The listing builds one solid part. Answer for the finished solid, in the listing's coordinates (mm). A direction names the side the tool comes from. Round coordinates to 2 decimals unless told otherwise and drop trailing zeros. Write each loop counter-clockwise with the first axis right and the second up, starting at its lowest first coordinate (ties: lowest second). Pieces come first, ordered by that corner, then holes. Notation, with made-up numbers: (21.25, 32.25) - (45.25, 32.25) arc R5 ccw to (45.25, 38.25) - close; hole circle Ø2 at (48.5, 73). An arc over 180 degrees is marked (long way). Answer as CSV lines item,"result". Start each with the question number.
Item 1: Which of the six approach directions +Z, -Z, +X, -X, +Y, -Y give full straight-line access (tool end or side, diameter ignored) to faces 1 (the cylindrical face through (40.9, 15.5, 3)), 2 (the flat face through (18, -27.5, 3)), 3 (the cylindrical face through (180.9, -15.5, 3))?
Item 2: A cutting plane is placed at A-A on z = 3.8. State how many separate pieces and enclosed holes the cut face has, and give its area (3 significant figures).
Item 3: A flat-ended cylindrical pin translates along its axis: pin 1 (2 mm diameter, centred on x = 226, y = 0, fed in from -Z). Find the tip coordinate at first contact, or state that the pin passes through.
Item 4: A cutting plane is placed at B-B on x = 148.5. Determine the outline of the cut face in (y, z), and give its area (3 significant figures).
Item 5: Straight lines are drawn through the part: line 1 along Y through (x, z) = (15, 3.35); line 2 along Y through (x, z) = (38.5, 4.9); line 3 along X through (y, z) = (-11.5, 5.25). For each, find the intervals that lie inside material, in ascending order. Write a range as [from, to].
```python
from build123d import *

# Parameters (mm, degrees)
SKETCH1_W           = 240
SKETCH1_H           = 25
SKETCH1_R           = 1.75
BOSS_EXTRUDE1_DEPTH = 6
SKETCH2_W           = 50
SKETCH2_H           = 10
BOSS_EXTRUDE2_DEPTH = 6
SKETCH3_W           = 140
SKETCH3_H           = 4
CUT_EXTRUDE1_DEPTH  = 235.693949645
SKETCH4_R           = 2.75
CUT_EXTRUDE2_DEPTH  = 235.693949645
FILLET1_R           = 7


with BuildPart() as part:
    # Sketch1 → Boss-Extrude1 (new body)
    with BuildSketch(Plane.XY):
        with Locations((113, -5)):
            Rectangle(SKETCH1_W, SKETCH1_H)
        Circle(SKETCH1_R, mode=Mode.SUBTRACT)
        with Locations((226, 0)):
            Circle(SKETCH1_R, mode=Mode.SUBTRACT)
        with Locations((15, 0)):
            Circle(SKETCH1_R, mode=Mode.SUBTRACT)
        with Locations((0, -10)):
            Circle(SKETCH1_R, mode=Mode.SUBTRACT)
        with Locations((15, -10)):
            Circle(SKETCH1_R, mode=Mode.SUBTRACT)
        with Locations((211, 0)):
            Circle(SKETCH1_R, mode=Mode.SUBTRACT)
        with Locations((211, -10)):
            Circle(SKETCH1_R, mode=Mode.SUBTRACT)
        with Locations((226, -10)):
            Circle(SKETCH1_R, mode=Mode.SUBTRACT)
        with Locations((183, -5)):
            Circle(SKETCH1_R, mode=Mode.SUBTRACT)
        with Locations((163, -5)):
            Circle(SKETCH1_R, mode=Mode.SUBTRACT)
        with Locations((143, -5)):
            Circle(SKETCH1_R, mode=Mode.SUBTRACT)
        with Locations((123, -5)):
            Circle(SKETCH1_R, mode=Mode.SUBTRACT)
        with Locations((103, -5)):
            Circle(SKETCH1_R, mode=Mode.SUBTRACT)
        with Locations((83, -5)):
            Circle(SKETCH1_R, mode=Mode.SUBTRACT)
        with Locations((63, -5)):
            Circle(SKETCH1_R, mode=Mode.SUBTRACT)
        with Locations((43, -5)):
            Circle(SKETCH1_R, mode=Mode.SUBTRACT)
    extrude(amount=BOSS_EXTRUDE1_DEPTH)

    # Sketch2 → Boss-Extrude2 (add)
    with BuildSketch(Plane.XY.offset(6)):
        with Locations((18, -22.5)):
            Rectangle(SKETCH2_W, SKETCH2_H)
        with Locations((18, 12.5)):
            Rectangle(SKETCH2_W, SKETCH2_H)
        with Locations((208, 12.5)):
            Rectangle(SKETCH2_W, SKETCH2_H)
        with Locations((208, -22.5)):
            Rectangle(SKETCH2_W, SKETCH2_H)
    extrude(amount=-BOSS_EXTRUDE2_DEPTH)

    # Sketch3 → Cut-Extrude1 (cut, through all)
    with BuildSketch(Plane(origin=(0, 0, 0), x_dir=(-1, 0, 0), z_dir=(0, 0, -1))):
        with Locations((-113, 5.5)):
            Rectangle(SKETCH3_W, SKETCH3_H)
        with Locations((-113, -15.5)):
            Rectangle(SKETCH3_W, SKETCH3_H)
    extrude(amount=-CUT_EXTRUDE1_DEPTH, mode=Mode.SUBTRACT)

    # Sketch4 → Cut-Extrude2 (cut, through all)
    with BuildSketch(Plane.XY.offset(6)):
        with Locations((36, -20)):
            Circle(SKETCH4_R)
        with Locations(Location((36, 10, 0), (0, 0, 180))):
            Circle(SKETCH4_R)
        with Locations((190, 10)):
            Circle(SKETCH4_R)
        with Locations(Location((190, -20, 0), (0, 0, 180))):
            Circle(SKETCH4_R)
    extrude(amount=-CUT_EXTRUDE2_DEPTH, mode=Mode.SUBTRACT)

    # Fillet1
    fillet1_edges = [part.edges().sort_by_distance(p)[0] for p in [
        (183, 3.5, 3),
        (183, 17.5, 3),
        (233, 17.5, 3),
        (233, -27.5, 3),
        (183, -13.5, 3),
        (183, -27.5, 3),
        (43, -13.5, 3),
        (43, 3.5, 3),
        (43, 17.5, 3),
        (-7, 17.5, 3),
        (43, -27.5, 3),
        (-7, -27.5, 3),
    ]]
    fillet(fillet1_edges, radius=FILLET1_R - 0.0001)  # a hair under: the kernel refuses the full size


solid = part.part
```
Geometry says:
1,face 1,"+Z, -Z, +Y"
1,face 2,"+Z, -Z, +X, -X, -Y"
1,face 3,"+Z, -Z, -Y"
2,separate pieces,"1"
2,enclosed holes,"20"
2,area,"6,590 mm^2"
3,pin 1,"passes through"
4,outline,"(-13.5, 0) - (3.5, 0) - (3.5, 6) - (-13.5, 6) - close"
4,area,"102 mm^2"
5,line 1,"y = [-27.5, -11.75], [-8.25, -1.75], [1.75, 17.5]"
5,line 2,"y = [-27.04, -21.15], [-18.85, 8.85], [11.15, 17.04]"
5,line 3,"x = [-7, -0.9], [0.9, 14.1], [15.9, 210.1], [211.9, 225.1], [226.9, 233]"
